Autodesk Inventor part; units mm, degrees
ref_plane "Work Plane1" through (10.2954, 3.175, -3.175) normal (0.7071, 0.7071, 0) x (-0.7071, 0.7071, 0)
ref_plane "YZ Plane" through (0, 0, 0) normal (1, 0, 0) x (0, 1, 0)
ref_plane "XZ Plane" through (0, 0, 0) normal (0, 1, 0) x (-1, 0, 0)
sketch "Sketch1" plane through (0, 0, 0) normal (0, 1, 0) x (-1, 0, 0)
  circle A0 centre (0, 0) radius 3.175
  dimension "d0" = 6.35
extrude "Extrusion1" add sketch "Sketch1" along normal blind 22.225
pattern_circular "Circular Pattern1" count 4 over 360 about axis through (0, 0, -10) along (0, 0, 1) of "Extrusion1"
sketch "Sketch2" plane through (0, 0, 0) normal (0, 0, 1) x (1, 0, 0)
  line L0 (0, 0) -> (3.175, -3.175)
  circle A0 centre (0, 0) radius 9.525
  dimension "d6" = 19.05
extrude "Extrusion2" add sketch "Sketch2" along normal mid plane 6.35
sketch "Sketch3" plane through (0, 0, -3.175) normal (0, 0, -1) x (-1, 0, 0)
  point P0 (0, 0)
  point P1 (0, 0)
hole "Hole1" at (0, 0, -3.175) direction (0, 0, 1) diameter 6.858 depth 25.4 tip angle 118
sketch "Sketch4" plane through (0, 0, -3.175) normal (0, 0, -1) x (-1, 0, 0)
  line L0 (-3.175, 8.9803) -> (-3.175, 22.225)
  line L1 (-22.225, 3.175) -> (-8.9803, 3.175)
  arc A0 (0, 9.525) -> (-9.525, 0) centre (0, 0) ccw
  line L2 (-10.2954, 3.175) -> (-3.175, 10.2954)
  point P0 (0, 0)
  dimension "d16" = 45
ref_plane "Work Plane1" through (10.2954, 3.175, -3.175) normal (0.7071, 0.7071, 0) x (-0.7071, 0.7071, 0)
sketch "Sketch5" plane through (10.2954, 3.175, -3.175) normal (0.7071, 0.7071, 0) x (-0.7071, 0.7071, 0)
  point P0 (5.0349, 3.175)
  point P1 (5.0349, 3.175)
properties part number "SweeperHub"
CAD build for the part. Positions are in the model's coordinates, mm. A direction names the side the tool comes from. Round coordinates to 2 decimals unless told otherwise and drop trailing zeros. Order: outer loops, then holes, each group sorted by start corner. A loop starts at its lowest first (then second) coordinate and runs counter-clockwise, first axis right, second up. Notation, with made-up numbers: (11.25, 51.25) -> (53.25, 51.25) arc R32 cw to (53.25, 82.25) -> close; hole circle Ø3 at (-23, 30). An arc over 180 degrees is marked (long way). Write item = value, one per line.
(1) Drill centre lines: L1, parallel to Y at x = 0, z = 0 (3 decimals); L2, parallel to Y at x = 1.5, z = -1 (3 decimals). Where is each one in solid material? Low to high.
Answers follow:
L1 = -22.225 to -3.429, 3.429 to 22.225
L2 = -22.225 to -3.084, 3.084 to 22.225
(2) Cut at B-B (y = 2). Write the cut outline in (x, z) (3 decimals), plus the area to 3 significant figures.
Answers follow:
outline = (-22.225, -2.466) -> (-9.313, -2.466) -> (-9.313, -3.175) -> (-2.785, -3.175) -> (-2.785, 3.175) -> (-9.313, 3.175) -> (-9.313, 2.466) -> (-22.225, 2.466) -> close; (2.785, -3.175) -> (9.313, -3.175) -> (9.313, -2.466) -> (22.225, -2.466) -> (22.225, 2.466) -> (9.313, 2.466) -> (9.313, 3.175) -> (2.785, 3.175) -> close
area = 210 mm²
(3) 3-axis set-ups, long thin cutter, end or side, ignore diameter. For faces 4 (the cylindrical face through (0.69, 15.7, -3.1)), 5 (the cylindrical face through (-15.51, 0.69, 3.1)), 6 (the flat face through (4, 0, 3.175)): which of +Z, -Z, +X, -X, +Y, -Y reach the whole face in a straight line?
Answers follow:
face_4 = +Y
face_5 = -X
face_6 = +Z, +X, -X, +Y, -Y
(4) Pull direction Y, two halves, no side cores. Call faces 1 (the cylindrical face through (15.51, -0.69, 3.1)), 2 (the cylindrical face through (3.35, -0.74, 0.04)), 3 (the cylindrical face through (-0.69, -15.51, 3.1)): +Y half, -Y half, draft (parallel to the pull), parting line (faces both ways), or undercut.
Answers follow:
face_1 = parting line
face_2 = undercut
face_3 = draft
(5) Flat gauge pins, fed straight in: P1, Ø2, axis at x = -7.5, z = 2.5, coming from the -Y side; P2, Ø3, axis at y = -14.5, z = 2, coming from the +X side; P3, Ø8, axis at x = 11, y = 10.5, coming from the +Z side; P4, Ø1.5, axis at y = 11.5, z = 0.5, coming from the +X side (3 decimals). Where does each tip first touch, or does it go through?
Answers follow:
P1 = -6.96
P2 = 3.14
P3 = through
P4 = 3.175
(6) Cut at A-A (z = 0). Write the cut outline in (x, y) (3 decimals).
Answers follow:
outline = (-22.225, -3.175) -> (-8.98, -3.175) arc R9.525 ccw to (-3.175, -8.98) -> (-3.175, -22.225) -> (3.175, -22.225) -> (3.175, -8.98) arc R9.525 ccw to (8.98, -3.175) -> (22.225, -3.175) -> (22.225, 3.175) -> (8.98, 3.175) arc R9.525 ccw to (3.175, 8.98) -> (3.175, 22.225) -> (-3.175, 22.225) -> (-3.175, 8.98) arc R9.525 ccw to (-8.98, 3.175) -> (-22.225, 3.175) -> close; hole circle Ø6.858 at (0, 0)
(7) Cut at C-C (x = 13). Write the cut outline in (y, z) (3 decimals), plus the area to 3 significant figures.
Answers follow:
outline = circle Ø6.35 at (0, 0)
area = 31.7 mm²
